Could you check a few things on this model? Use its own coordinates, in mm. Face numbers are marked on the shaded views. A direction names the side the tool comes from. Coordinates: 2 decimals unless noted, no trailing zeros. Write each loop counter-clockwise with the first axis right and the second up, starting at its lowest first coordinate (ties: lowest second). Pieces come first, ordered by that corner, then holes.
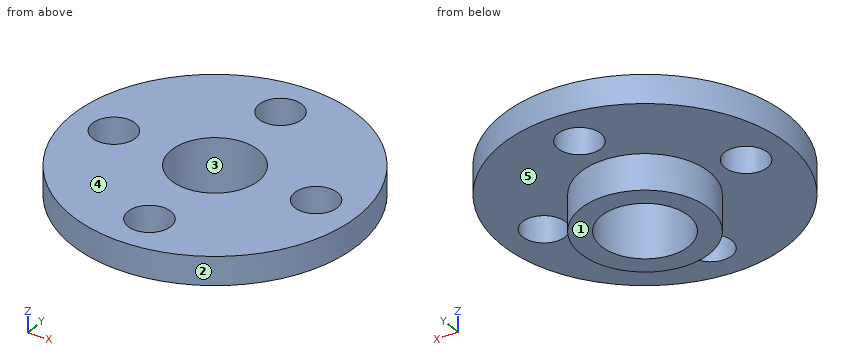
```python
from build123d import *

# Parameters (mm, degrees)
METAL_DISC_OD20_THICKNESS2_PROFILE_R       = 10
METAL_DISC_OD20_THICKNESS2_PROFILE_R_2     = 3.05
METAL_DISC_OD20_THICKNESS2_DEPTH           = 2
PURCHASED_25T_HUB_ENVELOPE_OD9_START       = -2.5
PURCHASED_25T_HUB_ENVELOPE_OD9_PROFILE_R   = 4.5
PURCHASED_25T_HUB_ENVELOPE_OD9_PROFILE_R_2 = 3.05
PURCHASED_25T_HUB_ENVELOPE_OD9_DEPTH       = 2.5
FOUR_M3_TAPPED_HOLE_ENVELOPES_PCD14_START  = -50
FOUR_M3_TAPPED_HOLE_ENVELOPES_PCD14_PROF_R = 1.5
FOUR_M3_TAPPED_HOLE_ENVELOPES_PCD14_DEPTH  = 65.361406616


with BuildPart() as part:
    # Metal_disc_OD20_thickness2_profile → Metal_disc_OD20_thickness2 (new body)
    with BuildSketch(Plane.XY):
        Circle(METAL_DISC_OD20_THICKNESS2_PROFILE_R)
        Circle(METAL_DISC_OD20_THICKNESS2_PROFILE_R_2, mode=Mode.SUBTRACT)
    extrude(amount=METAL_DISC_OD20_THICKNESS2_DEPTH)

    # Purchased_25T_hub_envelope_OD9_profile → Purchased_25T_hub_envelope_OD9 (add)
    with BuildSketch(Plane.XY.offset(PURCHASED_25T_HUB_ENVELOPE_OD9_START)):
        Circle(PURCHASED_25T_HUB_ENVELOPE_OD9_PROFILE_R)
        Circle(PURCHASED_25T_HUB_ENVELOPE_OD9_PROFILE_R_2, mode=Mode.SUBTRACT)
    extrude(amount=PURCHASED_25T_HUB_ENVELOPE_OD9_DEPTH)

    # Four_M3_tapped_hole_envelopes_PCD14_profile → Four_M3_tapped_hole_envelopes_PCD14 (cut, through all)
    with BuildSketch(Plane.XY.offset(FOUR_M3_TAPPED_HOLE_ENVELOPES_PCD14_START)):
        with Locations((-7, 0)):
            Circle(FOUR_M3_TAPPED_HOLE_ENVELOPES_PCD14_PROF_R)
        with Locations((7, 0)):
            Circle(FOUR_M3_TAPPED_HOLE_ENVELOPES_PCD14_PROF_R)
        with Locations((0, -7)):
            Circle(FOUR_M3_TAPPED_HOLE_ENVELOPES_PCD14_PROF_R)
        with Locations((0, 7)):
            Circle(FOUR_M3_TAPPED_HOLE_ENVELOPES_PCD14_PROF_R)
    extrude(amount=FOUR_M3_TAPPED_HOLE_ENVELOPES_PCD14_DEPTH, mode=Mode.SUBTRACT)


solid = part.part
```
1. If we mould it in two halves opening along X, with no side actions, what happens to the marked faces 1, 2 and 3? For each: pulls with the +X half, pulls with the -X half, needs draft (parallel to the pull), parting line crosses it, or undercut.
Verdict:
face 1: needs draft
face 2: parting line crosses it
face 3: undercut
2. I want a section at C-C on z = 1.75. Please give me the cut outline in (x, y), plus the area to 3 significant figures.
Verdict:
outline: circle Ø20 at (0, 0); hole circle Ø3 at (-7, 0); hole circle Ø6.1 at (0, 0); hole circle Ø3 at (0, -7); hole circle Ø3 at (0, 7); hole circle Ø3 at (7, 0)
area: 257 mm2
3. For pin 1 (1 mm diameter, centred on y = 1.5, z = 1, fed in from -X); pin 2 (3.5 mm diameter, centred on x = -7, y = 0, fed in from -Z); pin 3 (2.5 mm diameter, centred on x = 0, y = 7, fed in from -Z); pin 4 (1 mm diameter, centred on x = -2, z = -1, fed in from +Y), each with a flat end and sliding along its axis, tell me the tip position at first contact or that it passes through.
Verdict:
pin 1: stops at x = -9.95
pin 2: stops at z = 0
pin 3: passes through
pin 4: stops at y = 4.24
4. I want a section at A-A on y = 0. Please give me the cut outline in (x, z), plus the area to 4 significant figures.
Verdict:
outline: (-10, 0) - (-8.5, 0) - (-8.5, 2) - (-10, 2) - close; (-5.5, 0) - (-4.5, 0) - (-4.5, -2.5) - (-3.05, -2.5) - (-3.05, 2) - (-5.5, 2) - close; (3.05, -2.5) - (4.5, -2.5) - (4.5, 0) - (5.5, 0) - (5.5, 2) - (3.05, 2) - close; (8.5, 0) - (10, 0) - (10, 2) - (8.5, 2) - close
area: 23.05 mm2
5. On a 3-axis mill with a long thin cutter (end or side, diameter ignored), from which of +Z, -Z, +X, -X, +Y, -Y can I reach the whole of each face in a straight line? I mean the marked faces 4 and 5. Say none if no direction works.
Verdict:
face 4: +Z, +X, -X, +Y, -Y
face 5: -Z
6. Please list where these lines run through material, in increasing order: line 1 along Z through (x, y) = (5.5, -7.5); line 2 along Y through (x, z) = (-0.75, -0.25); line 3 along Y through (x, z) = (0.5, -0.2).
Verdict:
line 1: z = 0 to 2
line 2: y = -4.44 to -2.96, 2.96 to 4.44
line 3: y = -4.47 to -3.01, 3.01 to 4.47
7. I want a section at D-D on y = -7. Please give me the cut outline in (x, z), plus the area to 3 significant figures.
Verdict:
outline: (-7.14, 0) - (-1.5, 0) - (-1.5, 2) - (-7.14, 2) - close; (1.5, 0) - (7.14, 0) - (7.14, 2) - (1.5, 2) - close
area: 22.6 mm2
